from build123d import *

# Parameters (mm, degrees)
SKETCH_2_R          = 3
SKETCH_3_R          = 25
CUT_EXTRUDE_1_DEPTH = 5
SKETCH_4_R          = 35
CUT_EXTRUDE_2_DEPTH = 10


with BuildPart() as part:
    # ｽｹｯﾁ2 → 回転1 (revolve)
    with BuildSketch(Plane.XY, mode=Mode.PRIVATE) as revolve_1_sk:
        with Locations((27.5, 0)):
            Circle(SKETCH_2_R)
    revolve(revolve_1_sk.sketch.rotate(Axis((0, 0, 0), (0, 1, 0)), 90), axis=Axis((0, 0, 0), (0, 1, 0)))

    # ｽｹｯﾁ3 → ｶｯﾄ - 押し出し1 (cut, symmetric)
    with BuildSketch(Plane(origin=(0, 0, 0), x_dir=(1, 0, 0), z_dir=(0, 1, 0))):
        with Locations(Location((0, 0, 0), (0, 0, 90))):
            Circle(SKETCH_3_R)
    extrude(amount=CUT_EXTRUDE_1_DEPTH, both=True, mode=Mode.SUBTRACT)

    # ｽｹｯﾁ4 → ｶｯﾄ - 押し出し2 (cut)
    with BuildSketch(Plane(origin=(0, 2.5, 0), x_dir=(1, 0, 0), z_dir=(0, 1, 0))):
        Circle(SKETCH_4_R)
    extrude(amount=CUT_EXTRUDE_2_DEPTH, mode=Mode.SUBTRACT)


solid = part.part
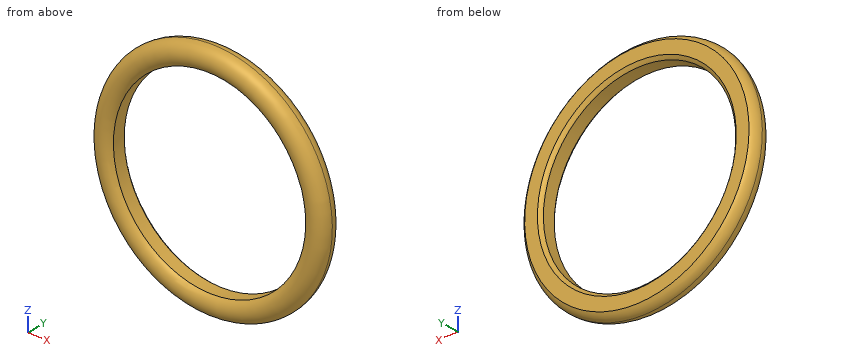
Verification items for the finished model (mm, model axes). Coordinates: 2 decimals unless noted, no trailing zeros. Order: outer loops, then holes, each group sorted by start corner. A loop starts at its lowest first (then second) coordinate and runs counter-clockwise, first axis right, second up.
1. Scan lines: line 1 (X direction, y = -0.1, z = 0); line 2 (X direction, y = -1.2, z = -5); line 3 (Z direction, x = -0.5, y = 1.8). Record each from-to range of solid material in increasing order.
Results found:
line 1: x = -30.5 to -25, 25 to 30.5
line 2: x = -29.83 to -24.49, 24.49 to 29.83
line 3: z = -29.9 to -25.1, 25.1 to 29.9
2. Sectioned sample at B-B, the plane x = 0. Record the cut outline in (y, z).
Results found:
outline: (-1.66, -25) arc R3 ccw (long way) to (2.5, -29.16) - (2.5, -25.84) arc R3 ccw to (1.66, -25) - close; (-1.66, 25) - (1.66, 25) arc R3 ccw to (2.5, 25.84) - (2.5, 29.16) arc R3 ccw (long way) to start
3. Go/stop test with flat-tipped pins: pin 1 Ø3 at (x, z) = (19, -12) entering from +Y; pin 2 Ø2 at (y, z) = (-1.5, -1.5) entering from +X; pin 3 Ø2 at (x, y) = (17.5, 0) entering from -Z; pin 4 Ø1 at (x, y) = (18, 1) entering from -Z. Record where each tip stops, or that it passes through.
Results found:
pin 1: passes through
pin 2: stops at x = 30.43
pin 3: stops at z = -25.65
pin 4: stops at z = -24.82
4. Sectioned sample at A-A, the plane z = 0. Record the cut outline in (x, y).
Results found:
outline: (-29.16, 2.5) arc R3 ccw (long way) to (-25, -1.66) - (-25, 1.66) arc R3 ccw to (-25.84, 2.5) - close; (25, -1.66) arc R3 ccw (long way) to (29.16, 2.5) - (25.84, 2.5) arc R3 ccw to (25, 1.66) - close
